```python
from build123d import *

# Parameters (mm, degrees)
SKETCH1_R           = 1.5
SKETCH1_R_2         = 2
SKETCH1_R_3         = 1.45
BOSS_EXTRUDE1_DEPTH = 2
CUT_EXTRUDE1_DEPTH  = 2
FILLET1_R           = 3
SKETCH3_R           = 1.5
CUT_EXTRUDE2_DEPTH  = 10
SKETCH_1_W          = 11.141106223
SKETCH_1_H          = 2.064068387
CUT_EXTRUDE_1_DEPTH = 10
SKETCH_2_R          = 4
CUT_EXTRUDE_2_DEPTH = 96.448488805
FILLET2_R           = 2
SKETCH4_R           = 1
CUT_EXTRUDE3_DEPTH  = 10
SKETCH5_W           = 11.82747082
SKETCH5_H           = 19.50302412
CUT_EXTRUDE4_DEPTH  = 10
FILLET3_R           = 1


with BuildPart() as part:
    # Sketch1 → Boss-Extrude1 (new body)
    with BuildSketch(Plane(origin=(0, 0, 0), x_dir=(1, 0, 0), z_dir=(0, 1, 0))):
        with BuildLine():
            Line((54.869224403, -12.305407816), (44.089868135, -12.305407816))
            ThreePointArc((44.089868135, -12.305407816), (41.968547791, -11.42672816), (41.089868135, -9.305407816))
            Line((41.089868135, -9.305407816), (41.089868135, 2.471948803))
            ThreePointArc((41.089868135, 2.471948803), (41.968547791, 4.593269147), (44.089868135, 5.471948803))
            Line((44.089868135, 5.471948803), (54.869224403, 5.471948803))
            ThreePointArc((54.869224403, 5.471948803), (56.990544747, 6.35062846), (57.869224403, 8.471948803))
            Line((57.869224403, 8.471948803), (57.869224403, 17.375765412))
            ThreePointArc((57.869224403, 17.375765412), (58.74790406, 19.497085755), (60.869224403, 20.375765412))
            Line((60.869224403, 20.375765412), (78.389804663, 20.375765412))
            Line((78.389804663, 20.375765412), (78.389804663, 27.585770494))
            Line((78.389804663, 27.585770494), (58.389804663, 47.585770494))
            Line((58.389804663, 47.585770494), (20.979804663, 47.585770494))
            Line((20.979804663, 47.585770494), (9.812981375, 26.583270494))
            Line((9.812981375, 26.583270494), (-13.868656246, 26.583270494))
            Line((-13.868656246, 26.583270494), (-44.620364758, 26.583270494))
            Line((-44.620364758, 26.583270494), (-44.620364758, 5.471948803))
            Line((-44.620364758, 5.471948803), (-13.868656246, 5.471948803))
            Line((-13.868656246, 5.471948803), (-13.868656246, -11.444658054))
            Line((-13.868656246, -11.444658054), (-25.009762469, -11.444658054))
            Line((-25.009762469, -11.444658054), (-25.009762469, -23.143538054))
            Line((-25.009762469, -23.143538054), (-3.796559034, -38.143538054))
            Line((-3.796559034, -38.143538054), (8.464513563, -38.143538054))
            Line((8.464513563, -38.143538054), (20.979804663, -54.419229506))
            Line((20.979804663, -54.419229506), (58.389804663, -54.419229506))
            Line((58.389804663, -54.419229506), (78.389804663, -34.419229506))
            Line((78.389804663, -34.419229506), (78.389804663, -27.209224425))
            Line((78.389804663, -27.209224425), (60.869224403, -27.209224425))
            ThreePointArc((60.869224403, -27.209224425), (58.74790406, -26.330544768), (57.869224403, -24.209224425))
            Line((57.869224403, -24.209224425), (57.869224403, -15.305407816))
            ThreePointArc((57.869224403, -15.305407816), (56.990544747, -13.184087473), (54.869224403, -12.305407816))
        make_face()
        with Locations(Location((32.479804663, -41.294229506, 0), (0, 0, 270))):
            Circle(SKETCH1_R, mode=Mode.SUBTRACT)
        with Locations(Location((41.979804663, -33.294229506, 0), (0, 0, 270))):
            Circle(SKETCH1_R, mode=Mode.SUBTRACT)
        with Locations(Location((32.479804663, -25.294229506, 0), (0, 0, 270))):
            Circle(SKETCH1_R, mode=Mode.SUBTRACT)
        with Locations(Location((22.979804663, -33.294229506, 0), (0, 0, 270))):
            Circle(SKETCH1_R, mode=Mode.SUBTRACT)
        with Locations(Location((-10.194098263, 24.120202053, 0), (0, 0, 270))):
            Circle(SKETCH1_R, mode=Mode.SUBTRACT)
        with Locations(Location((-22.049699545, -18.984613762, 0), (0, 0, 270))):
            Circle(SKETCH1_R, mode=Mode.SUBTRACT)
        with Locations(Location((3.798471154, -34.419229506, 0), (0, 0, 270))):
            Circle(SKETCH1_R, mode=Mode.SUBTRACT)
        with Locations(Location((57.193929966, -50.345885936, 0), (0, 0, 270))):
            Circle(SKETCH1_R_2, mode=Mode.SUBTRACT)
        with Locations(Location((55.174344354, -17.159547773, 0), (0, 0, 270))):
            Circle(SKETCH1_R, mode=Mode.SUBTRACT)
        with Locations(Location((55.174344354, 10.32608876, 0), (0, 0, 270))):
            Circle(SKETCH1_R, mode=Mode.SUBTRACT)
        with Locations(Location((-10.866471131, 3.389008325, 0), (0, 0, 270))):
            Circle(SKETCH1_R_3, mode=Mode.SUBTRACT)
        with Locations(Location((-5.208623843, -3.610189063, 0), (0, 0, 270))):
            Circle(SKETCH1_R_3, mode=Mode.SUBTRACT)
        with Locations(Location((1.790573544, -9.268036351, 0), (0, 0, 270))):
            Circle(SKETCH1_R_3, mode=Mode.SUBTRACT)
        with Locations(Location((57.193929966, 43.512426923, 0), (0, 0, 90))):
            Circle(SKETCH1_R_2, mode=Mode.SUBTRACT)
        with Locations(Location((22.979804663, 26.460770494, 0), (0, 0, 90))):
            Circle(SKETCH1_R, mode=Mode.SUBTRACT)
        with Locations(Location((32.479804663, 18.460770494, 0), (0, 0, 90))):
            Circle(SKETCH1_R, mode=Mode.SUBTRACT)
        with Locations(Location((41.979804663, 26.460770494, 0), (0, 0, 90))):
            Circle(SKETCH1_R, mode=Mode.SUBTRACT)
        with Locations(Location((32.479804663, 34.460770494, 0), (0, 0, 90))):
            Circle(SKETCH1_R, mode=Mode.SUBTRACT)
        with BuildLine():
            Line((16.558909908, -4.425834893), (17.596504785, -0.553478093))
            ThreePointArc((17.596504785, -0.553478093), (17.431334664, 0.901622726), (16.318958433, 1.854103006))
            ThreePointArc((16.318958433, 1.854103006), (6.440151022, 8.038585802), (0.255668225, 17.917393213))
            ThreePointArc((0.255668225, 17.917393213), (-0.696812054, 19.029769444), (-2.151912873, 19.194939566))
            Line((-2.151912873, 19.194939566), (-6.024269674, 18.157344688))
            ThreePointArc((-6.024269674, 18.157344688), (-7.269100914, 17.170851095), (-7.402354016, 15.588126218))
            ThreePointArc((-7.402354016, 15.588126218), (0.783296772, 2.381731553), (13.989691438, -5.803919235))
            ThreePointArc((13.989691438, -5.803919235), (15.572416314, -5.670666133), (16.558909908, -4.425834893))
        make_face(mode=Mode.SUBTRACT)
    extrude(amount=BOSS_EXTRUDE1_DEPTH)

    # Sketch2 → Cut-Extrude1 (cut)
    with BuildSketch(Plane.XZ):
        with BuildLine():
            Line((-40.041862968, -8.700189144), (-20.041862968, -8.700189144))
            ThreePointArc((-20.041862968, -8.700189144), (-18.541862968, -10.200189144), (-20.041862968, -11.700189144))
            Line((-20.041862968, -11.700189144), (-40.041862968, -11.700189144))
            ThreePointArc((-40.041862968, -11.700189144), (-41.541862968, -10.200189144), (-40.041862968, -8.700189144))
        make_face()
        with BuildLine():
            Line((-40.041862968, -17.700189144), (-20.041862968, -17.700189144))
            ThreePointArc((-20.041862968, -17.700189144), (-18.541862968, -16.200189144), (-20.041862968, -14.700189144))
            Line((-20.041862968, -14.700189144), (-40.041862968, -14.700189144))
            ThreePointArc((-40.041862968, -14.700189144), (-41.541862968, -16.200189144), (-40.041862968, -17.700189144))
        make_face()
        with BuildLine():
            Line((-40.041862968, -23.700189144), (-20.041862968, -23.700189144))
            ThreePointArc((-20.041862968, -23.700189144), (-18.541862968, -22.200189144), (-20.041862968, -20.700189144))
            Line((-20.041862968, -20.700189144), (-40.041862968, -20.700189144))
            ThreePointArc((-40.041862968, -20.700189144), (-41.541862968, -22.200189144), (-40.041862968, -23.700189144))
        make_face()
    extrude(amount=-CUT_EXTRUDE1_DEPTH, mode=Mode.SUBTRACT)

    # Fillet1
    fillet1_edges = [part.edges().sort_by_distance(p)[0] for p in [
        (-44.620364758, 1, -5.471948803),
        (-44.620364758, 1, -26.583270494),
    ]]
    fillet(fillet1_edges, radius=FILLET1_R)

    # Sketch3 → Cut-Extrude2 (cut)
    with BuildSketch(Plane.XZ):
        with Locations(Location((37.394868442, -44.049147495, 0), (0, 0, 270))):
            Circle(SKETCH3_R)
        with Locations(Location((37.394868442, 50.882606508, 0), (0, 0, 270))):
            Circle(SKETCH3_R)
        with Locations(Location((73.927423247, 31.637693078, 0), (0, 0, 270))):
            Circle(SKETCH3_R)
        with Locations(Location((73.927423247, -24.804234066, 0), (0, 0, 270))):
            Circle(SKETCH3_R)
    extrude(amount=-CUT_EXTRUDE2_DEPTH, mode=Mode.SUBTRACT)

    # 草图1 → 切除-拉伸1 (cut)
    with BuildSketch(Plane.XZ):
        with Locations((-19.439209358, 12.476692248)):
            Rectangle(SKETCH_1_W, SKETCH_1_H)
    extrude(amount=-CUT_EXTRUDE_1_DEPTH, mode=Mode.SUBTRACT)

    # 草图2 → 切除-拉伸2 (cut, through all)
    with BuildSketch(Plane.XZ):
        with Locations(Location((13.601488823, 29.543202895, 0), (0, 0, 270))):
            Circle(SKETCH_2_R)
        with Locations(Location((22.351612258, -36.336152346, 0), (0, 0, 270))):
            Circle(SKETCH_2_R)
    extrude(amount=-CUT_EXTRUDE_2_DEPTH, mode=Mode.SUBTRACT)

    # Fillet2
    fillet2_edges = [part.edges().sort_by_distance(p)[0] for p in [
        (-25.009762469, 1, 13.508726441),
        (58.389804663, 1, -47.585770494),
        (78.389804663, 1, -27.585770494),
        (78.389804663, 1, -20.375765412),
        (78.389804663, 1, 27.209224425),
        (78.389804663, 1, 34.419229506),
        (58.389804663, 1, 54.419229506),
        (20.979804663, 1, 54.419229506),
        (8.464513563, 1, 38.143538054),
        (-3.796559034, 1, 38.143538054),
        (-25.009762469, 1, 23.143538054),
        (-13.868656246, 1, -5.471948803),
        (9.812981375, 1, -26.583270494),
        (20.979804663, 1, -47.585770494),
    ]]
    fillet(fillet2_edges, radius=FILLET2_R)

    # Sketch4 → Cut-Extrude3 (cut)
    with BuildSketch(Plane(origin=(0, 2, 0), x_dir=(1, 0, 0), z_dir=(0, 1, 0))):
        with Locations((-13.868656246, -13.508726441)):
            Circle(SKETCH4_R)
    extrude(amount=-CUT_EXTRUDE3_DEPTH, mode=Mode.SUBTRACT)

    # Sketch5 → Cut-Extrude4 (cut)
    with BuildSketch(Plane(origin=(0, 2, 0), x_dir=(1, 0, 0), z_dir=(0, 1, 0))):
        with Locations((-18.928899697, -4.279563257)):
            Rectangle(SKETCH5_W, SKETCH5_H)
    extrude(amount=-CUT_EXTRUDE4_DEPTH, mode=Mode.SUBTRACT)

    # Fillet3
    fillet3_edges = [part.edges().sort_by_distance(p)[0] for p in [
        (-13.015164287, 1, -5.471948803),
    ]]
    fillet(fillet3_edges, radius=FILLET3_R)


solid = part.part
```
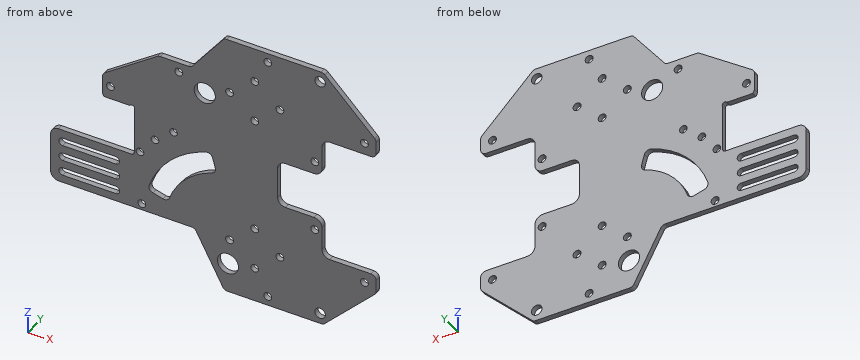
Can you work these out from the model? Positions are in its coordinate system, mm. Give positions to 0.01 mm unless a question says otherwise; leave off trailing zeros. Write each loop counter-clockwise with the first axis right and the second up, starting at its lowest first coordinate (ties: lowest second). Pieces come first, ordered by that corner, then holes. Notation, with made-up numbers: (43, -35) -> (53, -35) arc R26 ccw to (53, 1) -> close; hole circle Ø8 at (20.25, 73.25). An arc over 180 degrees is marked (long way). Write item = value, one per line.
(1) Suppose I cut it at D-D on y = 0.5. Count the separate pieces of the cut face and the enclosed holes in it, then the cut area to 3 significant figures.
Worked out:
separate_pieces = 1
enclosed_holes = 28
area = 6,680 mm^2
(2) Suppose I cut it at B-B on z = -39. Write out the boundary of the cut face in (x, y), then the cut area to 3 significant figures.
Worked out:
outline = (16.41, 0) -> (19.37, 0) -> (19.37, 2) -> (16.41, 2) -> close; (25.34, 0) -> (66.98, 0) -> (66.98, 2) -> (25.34, 2) -> close
area = 89.2 mm^2
(3) Suppose I cut it at C-C on x = 63. Write out the boundary of the cut face in (y, z).
Worked out:
outline = (0, -42.98) -> (2, -42.98) -> (2, -20.38) -> (0, -20.38) -> close; (0, 27.21) -> (2, 27.21) -> (2, 49.81) -> (0, 49.81) -> close
(4) I'm going to push flat-ended pins straight in: P1, Ø1, axis at x = -31, y = 0.5, coming from the +Z side; P2, Ø2.5, axis at x = -5.21, z = 3.61, coming from the -Y side; P3, Ø6.5, axis at x = 57.19, z = 50.35, coming from the -Y side. Where does each tip first touch, or does it pass through?
Worked out:
P1 = -5.47
P2 = through
P3 = 0
(5) Suppose I cut it at A-A on x = -35.5. Write out the boundary of the cut face in (y, z), then the cut area to 3 significant figures.
Worked out:
outline = (0, -26.58) -> (2, -26.58) -> (2, -23.7) -> (0, -23.7) -> close; (0, -20.7) -> (2, -20.7) -> (2, -17.7) -> (0, -17.7) -> close; (0, -14.7) -> (2, -14.7) -> (2, -11.7) -> (0, -11.7) -> close; (0, -8.7) -> (2, -8.7) -> (2, -5.47) -> (0, -5.47) -> close
area = 24.2 mm^2
(6) I need wall thicknesses on probe 1 along Z at (x, y) = (-37, 1.8); probe 2 along X at (y, z) = (1.35, 18.5); probe 3 along Z at (x, y) = (44.5, 0.2). Which ranges of each line are inside material? Lowest first, please. Write a range as from..to.
Worked out:
probe_1 = -26.58..-23.7, -20.7..-17.7, -14.7..-11.7, -8.7..-5.47
probe_2 = -25.01..-23.47, -20.63..54.5, 55.85..57.87
probe_3 = -47.59..-5.47, 12.31..54.42
